Part model, mm, in its own coordinate system. A direction names the side the tool comes from. Coordinates: 2 decimals unless noted, no trailing zeros. Write each loop counter-clockwise with the first axis right and the second up, starting at its lowest first coordinate (ties: lowest second). Pieces come first, ordered by that corner, then holes. Notation, with made-up numbers: (88.5, 83) - (138.5, 83) arc R7 cw to (138.5, 91) - close; hole circle Ø11 at (45.5, -33.75). An arc over 180 degrees is marked (long way). Write each question's results on one line, items separated by ' | '.
from build123d import *

# Parameters (mm, degrees)
SKETCH1_W           = 17.78
SKETCH1_H           = 20.32
BOSS_EXTRUDE1_DEPTH = 1.57
SKETCH2_R           = 2.797878481
BOSS_EXTRUDE2_DEPTH = 8.8
SKETCH3_R           = 1
CUT_EXTRUDE1_DEPTH  = 17.115138845


with BuildPart() as part:
    # Sketch1 → Boss-Extrude1 (new body)
    with BuildSketch(Plane(origin=(0, 0, 0), x_dir=(1, 0, 0), z_dir=(0, 1, 0))):
        Rectangle(SKETCH1_W, SKETCH1_H)
    extrude(amount=BOSS_EXTRUDE1_DEPTH)

    # Sketch2 → Boss-Extrude2 (add)
    with BuildSketch(Plane(origin=(0, 1.57, 0), x_dir=(1, 0, 0), z_dir=(0, 1, 0))):
        with Locations(Location((5.155350165, -3.588020089, 0), (0, 0, 270))):
            Circle(SKETCH2_R)
        with Locations(Location((-5.051725036, 0, 0), (0, 0, 270))):
            Circle(SKETCH2_R)
    extrude(amount=-BOSS_EXTRUDE2_DEPTH)

    # Sketch3 → Cut-Extrude1 (cut, through all)
    with BuildSketch(Plane(origin=(0, 1.57, 0), x_dir=(1, 0, 0), z_dir=(0, 1, 0))):
        with Locations(Location((-7.62, -8.89, 0), (0, 0, 270))):
            Circle(SKETCH3_R)
        with Locations(Location((7.62, 8.89, 0), (0, 0, 270))):
            Circle(SKETCH3_R)
    extrude(amount=-CUT_EXTRUDE1_DEPTH, mode=Mode.SUBTRACT)


solid = part.part
(1) 3-axis set-ups, long thin cutter, end or side, ignore diameter. For faces 5 (the cylindrical face through (5.278, -3.564, 0.793)), 6 (the flat face through (-5, -7.23, 0)): which of +Z, -Z, +X, -X, +Y, -Y reach the whole face in a straight line?
Return value:
face 5: -Y | face 6: +Z, -Z, +X, -X, -Y
(2) Saw through at B-B on z = 8.89. Write the cut outline in (x, y), then the cut area to 3 significant figures.
Return value:
outline: (-8.89, 0) - (-8.62, 0) - (-8.62, 1.57) - (-8.89, 1.57) - close; (-6.62, 0) - (8.89, 0) - (8.89, 1.57) - (-6.62, 1.57) - close | area: 24.8 mm^2
(3) Saw through at A-A on x = -7.62. Write the cut outline in (y, z).
Return value:
outline: (-7.23, -1.11) - (0, -1.11) - (0, -10.16) - (1.57, -10.16) - (1.57, 7.89) - (0, 7.89) - (0, 1.11) - (-7.23, 1.11) - close; (0, 9.89) - (1.57, 9.89) - (1.57, 10.16) - (0, 10.16) - close
(4) Wall check: line 1 (X direction, y = 0.6, z = -8.89); line 2 (Y direction, x = 7.5, z = 6); line 3 (X direction, y = 1.1, z = 8.89). Give the ranges that are in metal, low to high. Write a range as from..to.
Return value:
line 1: x = -8.89..6.62, 8.62..8.89 | line 2: y = 0..1.57 | line 3: x = -8.89..-8.62, -6.62..8.89
(5) Saw through at D-D on z = 0. Write the cut outline in (x, y).
Return value:
outline: (-8.89, 0) - (-7.85, 0) - (-7.85, -7.23) - (-2.25, -7.23) - (-2.25, 0) - (8.89, 0) - (8.89, 1.57) - (-8.89, 1.57) - close
(6) Two-plate mould, pull along X, no slides. Class faces 1 (the flat face through (8.89, 1, 0)), 2 (the flat face through (0, 1, 10.16)), 3 (the flat face through (-8.89, 1, 0)), 4 (the cylindrical face through (-7.534, -3.564, 1.291)): released by +X, released by -X, zero draft, split by the parting line, or undercut.
Return value:
face 1: released by +X | face 2: zero draft | face 3: released by -X | face 4: undercut
(7) Saw through at C-C on y = 0.25. Write the cut outline in (x, z).
Return value:
outline: (-8.89, -10.16) - (8.89, -10.16) - (8.89, 10.16) - (-8.89, 10.16) - close; hole circle Ø2 at (-7.62, 8.89); hole circle Ø2 at (7.62, -8.89)
(8) Flat gauge pins, fed straight in: P1, Ø3, axis at x = 3, y = -4.5, coming from the +Z side; P2, Ø2, axis at x = -6, y = -2, coming from the -Z side; P3, Ø1.5, axis at x = 0, z = -1, coming from the -Y side. Where does each tip first touch, or does it go through?
Return value:
P1: stops at z = 6.31 | P2: stops at z = -2.8 | P3: stops at y = 0
